Work out the finished part from the listing and answer in its coordinate system (mm). Give positions to 0.01 mm unless a question says otherwise; leave off trailing zeros. Loops run counter-clockwise (first coordinate to the right, second up) from the corner with the lowest first, then second, coordinate; pieces in that order, holes last.
```python
from build123d import *

# Parameters (mm, degrees)
SKETCH1_R           = 4.5
SKETCH1_R_2         = 45
BOSS_EXTRUDE1_DEPTH = 10


with BuildPart() as part:
    # Sketch1 → Boss-Extrude1 (new body)
    with BuildSketch(Plane.XY):
        with BuildLine():
            ThreePointArc((56.943478261, -7.980619246), (65.5, 0), (56.943478261, 7.980619246))
            ThreePointArc((56.943478261, 7.980619246), (49.796460718, 28.75), (35.383158136, 45.324189131))
            ThreePointArc((35.383158136, 45.324189131), (32.75, 56.724663948), (21.560320125, 53.304808377))
            ThreePointArc((21.560320125, 53.304808377), (0, 57.5), (-21.560320125, 53.304808377))
            ThreePointArc((-21.560320125, 53.304808377), (-32.75, 56.724663948), (-35.383158136, 45.324189131))
            ThreePointArc((-35.383158136, 45.324189131), (-49.796460718, 28.75), (-56.943478261, 7.980619246))
            ThreePointArc((-56.943478261, 7.980619246), (-65.5, 0), (-56.943478261, -7.980619246))
            ThreePointArc((-56.943478261, -7.980619246), (-48.897136106, -30.254257231), (-32.556086083, -47.39568819))
            ThreePointArc((-32.556086083, -47.39568819), (-31, -53.693575035), (-24.767826961, -51.89224169))
            ThreePointArc((-24.767826961, -51.89224169), (-1.752387282, -57.473290656), (21.560320125, -53.304808377))
            ThreePointArc((21.560320125, -53.304808377), (32.75, -56.724663948), (35.383158136, -45.324189131))
            ThreePointArc((35.383158136, -45.324189131), (49.796460718, -28.75), (56.943478261, -7.980619246))
        make_face()
        with Locations((57.5, 0)):
            Circle(SKETCH1_R, mode=Mode.SUBTRACT)
        with Locations((-57.5, 0)):
            Circle(SKETCH1_R, mode=Mode.SUBTRACT)
        with Locations((-28.75, 49.796460718)):
            Circle(SKETCH1_R, mode=Mode.SUBTRACT)
        with Locations((28.75, 49.796460718)):
            Circle(SKETCH1_R, mode=Mode.SUBTRACT)
        Circle(SKETCH1_R_2, mode=Mode.SUBTRACT)
        with Locations((28.75, -49.796460718)):
            Circle(SKETCH1_R, mode=Mode.SUBTRACT)
    extrude(amount=BOSS_EXTRUDE1_DEPTH)


solid = part.part
```
Q1. Section C-C on x = 28.75 is taken. Give the vertices of the cut face in (y, z), plus the area to 3 significant figures.
Q2. Section B-B on y = 0 is taken. Give the vertices of the cut face in (x, z).
Q3. Given pin 1 (2 mm diameter, centred on y = -27.5, z = 5.5, fed in from -X); pin 2 (6 mm diameter, centred on x = 4, z = 6, fed in from -Y); pin 3 (1.5 mm diameter, centred on y = 26, z = 2, fed in from +X), each flat-ended and moving along its own axis, determine where each tip first touches the part or whether it passes through.
Q4. Section D-D on z = 3 is taken. Give the vertices of the cut face in (x, y).
Q5. Determine the mould class of faces 1 (the face through (-65.498, 0.184, 4.93)), 2 (the face through (-15, -43, 10)), 3 (the face through (-53.208, 1.352, 4.93)) for opening direction Y: +Y half, -Y half, draft (parallel to the pull), parting line (faces both ways), or undercut.
Q6. Consider line 1 along Y through (x, z) = (28.75, 7.5); line 2 along X through (y, z) = (47, 2.75); line 3 along Y through (x, z) = (-28.75, 8). Determine where each line is inside the solid, lowest interval first.
Q7. Section A-A on x = 0 is taken. Give the vertices of the cut face in (y, z), plus the area to 3 significant figures.
Check result:
1. outline: (-57.8, 0) - (-54.3, 0) - (-54.3, 10) - (-57.8, 10) - close; (-45.3, 0) - (-34.62, 0) - (-34.62, 10) - (-45.3, 10) - close; (34.62, 0) - (45.3, 0) - (45.3, 10) - (34.62, 10) - close; (54.3, 0) - (57.8, 0) - (57.8, 10) - (54.3, 10) - close
1. area: 284 mm2
2. outline: (-65.5, 0) - (-62, 0) - (-62, 10) - (-65.5, 10) - close; (-53, 0) - (-45, 0) - (-45, 10) - (-53, 10) - close; (45, 0) - (53, 0) - (53, 10) - (45, 10) - close; (62, 0) - (65.5, 0) - (65.5, 10) - (62, 10) - close
3. pin 1: stops at x = -51.03
3. pin 2: stops at y = -57.49
3. pin 3: stops at x = 51.66
4. outline: (-56.94, -7.98) arc R57.5 ccw to (-32.56, -47.4) arc R4.5 ccw (long way) to (-24.77, -51.89) arc R57.5 ccw to (21.56, -53.3) arc R8 ccw (long way) to (35.38, -45.32) arc R57.5 ccw to (56.94, -7.98) arc R8 ccw (long way) to (56.94, 7.98) arc R57.5 ccw to (35.38, 45.32) arc R8 ccw (long way) to (21.56, 53.3) arc R57.5 ccw to (-21.56, 53.3) arc R8 ccw (long way) to (-35.38, 45.32) arc R57.5 ccw to (-56.94, 7.98) arc R8 ccw (long way) to start; hole circle Ø9 at (-57.5, 0); hole circle Ø90 at (0, 0); hole circle Ø9 at (-28.75, 49.8); hole circle Ø9 at (28.75, -49.8); hole circle Ø9 at (28.75, 49.8); hole circle Ø9 at (57.5, 0)
5. face 1: parting line
5. face 2: draft
5. face 3: undercut
6. line 1: y = -57.8 to -54.3, -45.3 to -34.62, 34.62 to 45.3, 54.3 to 57.8
6. line 2: x = -36.25 to -32.28, -25.22 to 25.22, 32.28 to 36.25
6. line 3: y = -54.3 to -34.62, 34.62 to 45.3, 54.3 to 57.8
7. outline: (-57.5, 0) - (-45, 0) - (-45, 10) - (-57.5, 10) - close; (45, 0) - (57.5, 0) - (57.5, 10) - (45, 10) - close
7. area: 250 mm2
